Can you work these out from the model? Positions are in its coordinate system, mm. A direction names the side the tool comes from. Give positions to 0.01 mm unless a question says otherwise; leave off trailing zeros. Loops run counter-clockwise (first coordinate to the right, second up) from the corner with the lowest first, then second, coordinate; pieces in that order, holes last. Notation, with made-up numbers: (22, -14.75) - (75, -14.75) arc R9 cw to (75, -1.75) - close; hole circle Ø4 at (5, 6.25). An arc over 180 degrees is marked (long way). Answer in a Markdown table with one row per item.
from build123d import *
from OCP.BRepFilletAPI import BRepFilletAPI_MakeChamfer

# Parameters (mm, degrees)
SKETCH_11_R         = 3.3
EXTRUDE_4_DEPTH     = 60
SKETCH_17_R         = 6
CUT_EXTRUDE_3_DEPTH = 19
SKETCH_18_R         = 6
CUT_EXTRUDE_4_DEPTH = 19
CUT_EXTRUDE_START   = -19
SKETCH_19_R         = 6
CUT_EXTRUDE_5_DEPTH = 19
SKETCH_21_R         = 6
CUT_EXTRUDE_6_DEPTH = 19
SKETCH_22_R         = 1.5
CUT_EXTRUDE_7_DEPTH = 100
SKETCH_28_R         = 3
EXTRUDE_5_DEPTH     = 1.5
CHAMFER_1_SIZE      = 1.5
CHAMFER_1_SIZE_2    = 0.5
SKETCH_29_R         = 1.5
CUT_EXTRUDE_9_DEPTH = 72.986055326


with BuildPart() as part:
    # 草图11 → 凸台-拉伸4 (new body)
    with BuildSketch(Plane(origin=(0, 0, 0), x_dir=(0, 0, -1), z_dir=(1, 0, 0))):
        with BuildLine():
            Line((-22.771084337, -3.256454389), (-22.771084337, -11.256454389))
            Line((-22.771084337, -11.256454389), (37.228915663, -11.256454389))
            Line((37.228915663, -11.256454389), (37.228915663, -3.256454389))
            Line((37.228915663, -3.256454389), (34.728915663, -3.256454389))
            ThreePointArc((34.728915663, -3.256454389), (28.728915663, 2.743545611), (22.728915663, -3.256454389))
            Line((22.728915663, -3.256454389), (-8.271084337, -3.256454389))
            ThreePointArc((-8.271084337, -3.256454389), (-14.271084337, 2.743545611), (-20.271084337, -3.256454389))
            Line((-20.271084337, -3.256454389), (-22.771084337, -3.256454389))
        make_face()
        with Locations((-14.271084337, -3.256454389)):
            Circle(SKETCH_11_R, mode=Mode.SUBTRACT)
        with Locations((28.728915663, -3.256454389)):
            Circle(SKETCH_11_R, mode=Mode.SUBTRACT)
    extrude(amount=-EXTRUDE_4_DEPTH)

    # 草图17 → 切除-拉伸3 (cut)
    with BuildSketch(Plane(origin=(-2.5, 0, 0), x_dir=(0, 0, -1), z_dir=(1, 0, 0))):
        with Locations((-14.271084337, -3.256454389)):
            Circle(SKETCH_17_R)
    extrude(amount=-CUT_EXTRUDE_3_DEPTH, mode=Mode.SUBTRACT)

    # 草图18 → 切除-拉伸4 (cut)
    with BuildSketch(Plane(origin=(-2.5, 0, 0), x_dir=(0, 0, -1), z_dir=(1, 0, 0))):
        with Locations((28.728915663, -3.256454389)):
            Circle(SKETCH_18_R)
    extrude(amount=-CUT_EXTRUDE_4_DEPTH, mode=Mode.SUBTRACT)

    # 草图19 → 切除-拉伸5 (cut)
    with BuildSketch(Plane.ZY.offset(57.5).offset(CUT_EXTRUDE_START)):
        with Locations((-28.728915663, -3.256454389)):
            Circle(SKETCH_19_R)
    extrude(amount=CUT_EXTRUDE_5_DEPTH, mode=Mode.SUBTRACT)

    # 草图21 → 切除-拉伸6 (cut)
    with BuildSketch(Plane.ZY.offset(57.5).offset(CUT_EXTRUDE_START)):
        with Locations((14.271084337, -3.256454389)):
            Circle(SKETCH_21_R)
    extrude(amount=CUT_EXTRUDE_6_DEPTH, mode=Mode.SUBTRACT)

    # 草图22 → 切除-拉伸7 (cut)
    with BuildSketch(Plane(origin=(0, -3.256454389, 0), x_dir=(1, 0, 0), z_dir=(0, 1, 0))):
        with Locations(Location((-30, 19.228915663, 0), (0, 0, 270))):
            Circle(SKETCH_22_R)
        with Locations(Location((-30, -4.771084337, 0), (0, 0, 270))):
            Circle(SKETCH_22_R)
        with Locations(Location((-18, 7.228915663, 0), (0, 0, 270))):
            Circle(SKETCH_22_R)
        with Locations(Location((-42, 7.228915663, 0), (0, 0, 270))):
            Circle(SKETCH_22_R)
        with Locations(Location((-19.87, 17.358915663, 0), (0, 0, 270))):
            Circle(SKETCH_22_R)
        with Locations(Location((-19.87, -2.901084337, 0), (0, 0, 270))):
            Circle(SKETCH_22_R)
        with Locations(Location((-40.15, -2.901084337, 0), (0, 0, 270))):
            Circle(SKETCH_22_R)
        with Locations(Location((-40.15, 17.358915663, 0), (0, 0, 270))):
            Circle(SKETCH_22_R)
    extrude(amount=-CUT_EXTRUDE_7_DEPTH, mode=Mode.SUBTRACT)

    # 草图28 → 凸台-拉伸5 (add)
    with BuildSketch(Plane.XZ.offset(11.256454389)):
        with Locations(Location((-19.87, 2.901084337, 0), (0, 0, 270))):
            Circle(SKETCH_28_R)
        with Locations(Location((-19.87, -17.358915663, 0), (0, 0, 270))):
            Circle(SKETCH_28_R)
        with Locations(Location((-40.15, -17.358915663, 0), (0, 0, 270))):
            Circle(SKETCH_28_R)
        with Locations(Location((-40.15, 2.901084337, 0), (0, 0, 270))):
            Circle(SKETCH_28_R)
    extrude(amount=EXTRUDE_5_DEPTH)

    # 倒角1
    chamfer_1_edges_1 = [part.edges().sort_by_distance(p)[0] for p in [
        (-19.87, -12.756454389, 5.901084337),
    ]]
    chamfer_1_side_1 = [part.faces().sort_by_distance(p)[0] for p in [
        (-19.87, -12.746454389, 5.901084337),
    ]]
    chamfer_1_edges_2 = [part.edges().sort_by_distance(p)[0] for p in [
        (-19.87, -12.756454389, -14.358915663),
    ]]
    chamfer_1_side_2 = [part.faces().sort_by_distance(p)[0] for p in [
        (-19.87, -12.746454389, -14.358915663),
    ]]
    chamfer_1_edges_3 = [part.edges().sort_by_distance(p)[0] for p in [
        (-40.15, -12.756454389, -14.358915663),
    ]]
    chamfer_1_side_3 = [part.faces().sort_by_distance(p)[0] for p in [
        (-40.15, -12.746454389, -14.358915663),
    ]]
    chamfer_1_edges_4 = [part.edges().sort_by_distance(p)[0] for p in [
        (-40.15, -12.756454389, 5.901084337),
    ]]
    chamfer_1_side_4 = [part.faces().sort_by_distance(p)[0] for p in [
        (-40.15, -12.746454389, 5.901084337),
    ]]
    chamfer_1 = BRepFilletAPI_MakeChamfer(part.part.solid().wrapped)
    for e in chamfer_1_edges_1:
        chamfer_1.Add(CHAMFER_1_SIZE - 0.0001, CHAMFER_1_SIZE_2 - 0.0001, e.wrapped, chamfer_1_side_1[0].wrapped)
    for e in chamfer_1_edges_2:
        chamfer_1.Add(CHAMFER_1_SIZE - 0.0001, CHAMFER_1_SIZE_2 - 0.0001, e.wrapped, chamfer_1_side_2[0].wrapped)
    for e in chamfer_1_edges_3:
        chamfer_1.Add(CHAMFER_1_SIZE - 0.0001, CHAMFER_1_SIZE_2 - 0.0001, e.wrapped, chamfer_1_side_3[0].wrapped)
    for e in chamfer_1_edges_4:
        chamfer_1.Add(CHAMFER_1_SIZE - 0.0001, CHAMFER_1_SIZE_2 - 0.0001, e.wrapped, chamfer_1_side_4[0].wrapped)
    add(Compound.cast(chamfer_1.Shape()), mode=Mode.REPLACE)  # a hair under: the kernel refuses the full size

    # 草图29 → 切除-拉伸9 (cut, through all)
    with BuildSketch(Plane(origin=(0, -11.256454389, 0), x_dir=(1, 0, 0), z_dir=(0, 1, 0))):
        with Locations(Location((-40.15, -2.901084337, 0), (0, 0, 270))):
            Circle(SKETCH_29_R)
        with Locations(Location((-40.15, 17.358915663, 0), (0, 0, 270))):
            Circle(SKETCH_29_R)
        with Locations(Location((-19.87, 17.358915663, 0), (0, 0, 270))):
            Circle(SKETCH_29_R)
        with Locations(Location((-19.87, -2.901084337, 0), (0, 0, 270))):
            Circle(SKETCH_29_R)
    extrude(amount=-CUT_EXTRUDE_9_DEPTH, mode=Mode.SUBTRACT)


solid = part.part
Q1. Imagine slicing it at D-D, the plane y = -5. Count the separate pieces of the cut face and the enclosed holes in it, and give its area (3 significant figures).
Checked values:
| item | result |
|---|---|
| separate pieces | 3 |
| enclosed holes | 8 |
| area | 2,420 mm² |
Q2. If I drill on line 1 (X direction, y = -7.25, z = -27); line 2 (Z direction, x = -40, y = -6); line 3 (Z direction, x = -19, y = -6.25), over which ranges is the centre line in solid material (lowest first)? Write a range as [from, to].
Checked values:
| item | result |
|---|---|
| line 1 | x = [-60, -57.5], [-38.5, -21.5], [-2.5, 0] |
| line 2 | z = [-37.23, -34.06], [-23.39, -18.85], [-15.87, 1.41], [4.39, 8.94], [19.61, 22.77] |
| line 3 | z = [-37.23, -33.93], [-23.53, -18.58], [-16.14, -8.35], [-6.11, 1.68], [4.12, 9.07], [19.47, 22.77] |
Q3. Imagine slicing it at B-B, the plane z = 13.5. Write out the boundary of the cut face in (x, y), and give its area (3 significant figures).
Checked values:
| item | result |
|---|---|
| outline | (-60, -11.26) - (0, -11.26) - (0, -6.47) - (-2.5, -6.47) - (-2.5, -9.21) - (-21.5, -9.21) - (-21.5, -6.47) - (-38.5, -6.47) - (-38.5, -9.21) - (-57.5, -9.21) - (-57.5, -6.47) - (-60, -6.47) - close; (-60, -0.05) - (-57.5, -0.05) - (-57.5, 2.69) - (-60, 2.69) - close; (-38.5, -0.05) - (-21.5, -0.05) - (-21.5, 2.69) - (-38.5, 2.69) - close; (-2.5, -0.05) - (0, -0.05) - (0, 2.69) - (-2.5, 2.69) - close |
| area | 244 mm² |
Q4. Imagine slicing it at C-C, the plane x = -14. Write out the boundary of the cut face in (y, z).
Checked values:
| item | result |
|---|---|
| outline | (-11.26, -37.23) - (-3.26, -37.23) - (-3.26, -34.73) arc R6 cw to (-3.26, -22.73) - (-3.26, 8.27) arc R6 cw to (-3.26, 20.27) - (-3.26, 22.77) - (-11.26, 22.77) - close |
Q5. For pin 1 (12 mm diameter, centred on x = -28.5, z = 6, fed in from +Y); pin 2 (4 mm diameter, centred on x = -18, z = -7.23, fed in from +Y); pin 3 (6 mm diameter, centred on x = -35.5, y = 0, fed in from -Z), each with a flat end and sliding along its axis, tell me the tip position at first contact or that it passes through.
Checked values:
| item | result |
|---|---|
| pin 1 | stops at y = 2.3 |
| pin 2 | stops at y = -3.26 |
| pin 3 | stops at z = -34.72 |
Q6. Imagine slicing it at A-A, the plane x = -30. Write out the boundary of the cut face in (y, z), and give its area (3 significant figures).
Checked values:
| item | result |
|---|---|
| outline | (-11.26, -37.23) - (-3.26, -37.23) - (-3.26, -34.73) arc R6 ccw to (-3.26, -22.73) - (-3.26, -20.73) - (-11.26, -20.73) - close; (-11.26, -17.73) - (-3.26, -17.73) - (-3.26, 3.27) - (-11.26, 3.27) - close; (-11.26, 6.27) - (-3.26, 6.27) - (-3.26, 8.27) arc R6 ccw to (-3.26, 20.27) - (-3.26, 22.77) - (-11.26, 22.77) - close; hole circle Ø6.6 at (-3.26, -28.73); hole circle Ø6.6 at (-3.26, 14.27) |
| area | 477 mm² |
Q7. If we mould it in two halves opening along X, with no side actions, what happens to faces 3 (the face through (-29.881, -3.111, -25.432)), 4 (the face through (-2.5, -6, 12))? For each: released by +X, released by -X, zero draft, split by the parting line, or undercut.
Checked values:
| item | result |
|---|---|
| face 3 | zero draft |
| face 4 | undercut |
Q8. On a 3-axis mill with a long thin cutter (end or side, diameter ignored), from which of +Z, -Z, +X, -X, +Y, -Y can I reach the whole of each face in a straight line? I mean faces 1 (the face through (-30, -7, 22.771)), 2 (the face through (-47.867, -9.255, 14.139)). Say none if no direction works.
Checked values:
| item | result |
|---|---|
| face 1 | +Z, +X, -X, +Y, -Y |
| face 2 | +Y |
